from build123d import *

# Parameters (mm, degrees)
SKETCH2_W           = 31.775877048
SKETCH2_H           = 56.6
SKETCH2_R           = 1.5
SKETCH2_W_2         = 21.775877048
SKETCH2_H_2         = 42.575877048
BOSS_EXTRUDE1_DEPTH = 7.5
SKETCH3_W           = 8
SKETCH3_H           = 2.5
BOSS_EXTRUDE2_DEPTH = 10
SKETCH4_R           = 1
CUT_EXTRUDE1_DEPTH  = 42.765016348
FILLET1_R           = 4
FILLET3_R           = 0.5
CHAMFER1_SIZE       = 0.1
CHAMFER2_SIZE       = 0.5


with BuildPart() as part:
    # Sketch2 → Boss-Extrude1 (new body)
    with BuildSketch(Plane.XY):
        Rectangle(SKETCH2_W, SKETCH2_H)
        with Locations((5, -24.889613301)):
            Circle(SKETCH2_R, mode=Mode.SUBTRACT)
        with Locations((-5, -24.889613301)):
            Circle(SKETCH2_R, mode=Mode.SUBTRACT)
        with Locations((5, 24.889613301)):
            Circle(SKETCH2_R, mode=Mode.SUBTRACT)
        with Locations((-5, 24.889613301)):
            Circle(SKETCH2_R, mode=Mode.SUBTRACT)
        Rectangle(SKETCH2_W_2, SKETCH2_H_2, mode=Mode.SUBTRACT)
    extrude(amount=BOSS_EXTRUDE1_DEPTH)

    # Sketch3 → Boss-Extrude2 (add)
    with BuildSketch(Plane.XZ.offset(28.3)):
        with Locations((0, 3.75)):
            Rectangle(SKETCH3_W, SKETCH3_H)
    extrude(amount=BOSS_EXTRUDE2_DEPTH)

    # Sketch4 → Cut-Extrude1 (cut, through all)
    with BuildSketch(Plane.XY.offset(5)):
        with Locations((0, -34.3)):
            Circle(SKETCH4_R)
    extrude(amount=-CUT_EXTRUDE1_DEPTH, mode=Mode.SUBTRACT)

    # Fillet1
    fillet1_edges = [part.edges().sort_by_distance(p)[0] for p in [
        (4, -38.3, 3.75),
        (-4, -38.3, 3.75),
    ]]
    fillet(fillet1_edges, radius=FILLET1_R - 0.0001)  # a hair under: the kernel refuses the full size

    # Fillet3
    fillet3_edges = [part.edges().sort_by_distance(p)[0] for p in [
        (-4, -28.3, 3.75),
        (0, -28.3, 2.5),
        (4, -28.3, 3.75),
        (0, -28.3, 5),
    ]]
    fillet(fillet3_edges, radius=FILLET3_R)

    # Chamfer1
    chamfer1_edges = [part.edges().sort_by_distance(p)[0] for p in [
        (-1, -34.3, 2.5),
        (-1, -34.3, 5),
    ]]
    chamfer(chamfer1_edges, length=CHAMFER1_SIZE)

    # Chamfer2
    chamfer2_edges = [part.edges().sort_by_distance(p)[0] for p in [
        (15.887938524, 0, 7.5),
        (0, 28.3, 7.5),
        (-15.887938524, 0, 7.5),
        (0, 28.3, 0),
        (15.887938524, 0, 0),
        (-15.887938524, 0, 0),
        (-15.887938524, 28.3, 3.75),
        (15.887938524, 28.3, 3.75),
    ]]
    chamfer(chamfer2_edges, length=CHAMFER2_SIZE)


solid = part.part
Source: CAD feature listing. Evaluate the final solid. Frame: model axes, mm. A direction names the side the tool comes from. Give positions to 0.01 mm unless a question says otherwise; leave off trailing zeros. Order: outer loops, then holes, each group sorted by start corner. A loop starts at its lowest first (then second) coordinate and runs counter-clockwise, first axis right, second up. Notation, with made-up numbers: (12, 85.25) -> (25, 85.25) arc R22 ccw to (25, 106.25) -> close; hole circle Ø10 at (84, 83.5). An arc over 180 degrees is marked (long way). Write item = value, one per line.
Q1. Cut plane A-A, the plane y = -19. Output: boundary loops of the cut face in (x, z).
Data:
outline = (-15.89, 0.5) -> (-15.39, 0) -> (-10.89, 0) -> (-10.89, 7.5) -> (-15.39, 7.5) -> (-15.89, 7) -> close; (10.89, 0) -> (15.39, 0) -> (15.89, 0.5) -> (15.89, 7) -> (15.39, 7.5) -> (10.89, 7.5) -> close
Q2. Cut plane C-C, the plane x = 5.5. Output: boundary loops of the cut face in (y, z), and give its area (3 significant figures).
Data:
outline = (-28.3, 0) -> (-26.3, 0) -> (-26.3, 7.5) -> (-28.3, 7.5) -> close; (-23.48, 0) -> (-21.29, 0) -> (-21.29, 7.5) -> (-23.48, 7.5) -> close; (21.29, 0) -> (23.48, 0) -> (23.48, 7.5) -> (21.29, 7.5) -> close; (26.3, 0) -> (27.8, 0) -> (28.3, 0.5) -> (28.3, 7) -> (27.8, 7.5) -> (26.3, 7.5) -> close
area = 62.5 mm^2
Q3. Pin query (flat end, axial travel): pin 1 (2.5 mm diameter, centred on x = 0, y = -34.3, fed in from -Z); pin 2 (2 mm diameter, centred on y = -31, z = 3.5, fed in from -X); pin 3 (4 mm diameter, centred on x = 0.5, y = -33, fed in from +Z). Return the tip coordinate at first contact, or that it passes through.
Data:
pin_1 = 2.5
pin_2 = -4
pin_3 = 5
Q4. Cut plane B-B, the plane x = 9.5. Output: boundary loops of the cut face in (y, z), and give its area (3 significant figures).
Data:
outline = (-28.3, 0) -> (-21.29, 0) -> (-21.29, 7.5) -> (-28.3, 7.5) -> close; (21.29, 0) -> (27.8, 0) -> (28.3, 0.5) -> (28.3, 7) -> (27.8, 7.5) -> (21.29, 7.5) -> close
area = 105 mm^2
Q5. Set-up query: faces 1 (the face through (0, -32, 5)), 2 (the face through (4, -32, 4)), 3 (the face through (10.888, 0, 4)), 4 (the face through (15.888, -1, 4)), 5 (the face through (-4, -32, 4)). Return all of +Z, -Z, +X, -X, +Y, -Y with unobstructed straight access to the full face (end or side cutting, diameter ignored); none if empty.
Data:
face_1 = +Z, +X, -X, -Y
face_2 = +Z, -Z, +X, -Y
face_3 = +Z, -Z
face_4 = +Z, -Z, +X, +Y, -Y
face_5 = +Z, -Z, -X, -Y
Q6. Cut plane D-D, the plane z = 3.25. State how many separate pieces and enclosed holes the cut face has, and give its area (3 significant figures).
Data:
separate_pieces = 1
enclosed_holes = 6
area = 913 mm^2
Q7. Pull-direction query (X, two-part tool) for faces 6 (the face through (2.859, -37.097, 3.768)), 7 (the face through (0, 28.3, 4)), 8 (the face through (-5.325, -26.354, 3.698)); classes: released by +X, released by -X, zero draft, split by the parting line, or undercut.
Data:
face_6 = released by +X
face_7 = zero draft
face_8 = undercut
Q8. Material intervals for line 1 (Y direction, x = 5, z = 5); line 2 (X direction, y = 25, z = 2.25); line 3 (Y direction, x = 0.5, z = 6.75), sorted ascending. Write a range as from..to.
Data:
line_1 = -28.3..-26.39, -23.39..-21.29, 21.29..23.39, 26.39..28.3
line_2 = -15.89..-6.5, -3.5..3.5, 6.5..15.89
line_3 = -28.3..-21.29, 21.29..28.3
